from build123d import *

# Parameters (mm, degrees)
SKETCH1_R           = 25.4
BOSS_EXTRUDE1_DEPTH = 3.175
SKETCH2_R           = 12.7
SKETCH2_R_2         = 4.7625
BOSS_EXTRUDE2_DEPTH = 25.4
SKETCH3_R           = 3.175
CUT_EXTRUDE1_DEPTH  = 29.575


with BuildPart() as part:
    # Sketch1 → Boss-Extrude1 (new body)
    with BuildSketch(Plane(origin=(0, 0, 0), x_dir=(1, 0, 0), z_dir=(0, 1, 0))):
        Circle(SKETCH1_R)
    extrude(amount=BOSS_EXTRUDE1_DEPTH)

    # Sketch2 → Boss-Extrude2 (add)
    with BuildSketch(Plane(origin=(0, 3.175, 0), x_dir=(1, 0, 0), z_dir=(0, 1, 0))):
        Circle(SKETCH2_R)
        Circle(SKETCH2_R_2, mode=Mode.SUBTRACT)
    extrude(amount=BOSS_EXTRUDE2_DEPTH)

    # Sketch3 → Cut-Extrude1 (cut, through all)
    with BuildSketch(Plane.XZ):
        with Locations((-12.7, 12.7)):
            Circle(SKETCH3_R)
        with Locations((12.7, 12.7)):
            Circle(SKETCH3_R)
        with Locations((12.7, -12.7)):
            Circle(SKETCH3_R)
        with Locations((-12.7, -12.7)):
            Circle(SKETCH3_R)
    extrude(amount=-CUT_EXTRUDE1_DEPTH, mode=Mode.SUBTRACT)


solid = part.part
Verification items for the finished model (mm, model axes). A direction names the side the tool comes from. Coordinates: 2 decimals unless noted, no trailing zeros. Order: outer loops, then holes, each group sorted by start corner. A loop starts at its lowest first (then second) coordinate and runs counter-clockwise, first axis right, second up. Notation, with made-up numbers: M 15,63 L 34,63 A5 cw 34,68 Z; hole C -26.5,66.25 d1. An arc over 180 degrees is marked long. One line per item, written item: value. Start each with the question number.
Item 1: Sectioned sample at B-B on z = 15. Record the cut outline in (x, y) (3 decimals).
Item 2: Depth check by flat-ended pin: P1, Ø1, axis at x = -5, y = 19, coming from the +Z side; P2, Ø3, axis at x = 8, y = 5.5, coming from the +Z side; P3, Ø5, axis at x = 12.7, z = -12.7, coming from the -Y side; P4, Ø4, axis at y = 23.5, z = 7, coming from the -X side. Enter the tip coordinate at first touch or a pass-through.
Item 3: Sectioned sample at C-C on x = 0. Record the cut outline in (y, z) (1 decimal).
Item 4: Sectioned sample at A-A on x = 12. Record the cut outline in (y, z) (3 decimals).
Item 5: Access from +Z, -Z, +X, -X, +Y, -Y to the whole of each face (thin tool, end or side, straight path). Record for faces 1 (the flat face through (0, 3.175, 0)), 2 (the flat face through (5, 28.575, 0)).
Item 6: Thickness scan on probe 1 along X at (y, z) = (19.5, 0); probe 2 along Z at (x, y) = (-12.7, 1.2) (3 decimals); probe 3 along X at (y, z) = (3, -10). Record the ranges inside material, lowest first.
Item 7: Sectioned sample at D-D on y = 10.5. Record the cut outline in (x, z) (1 decimal), then the cut area to 3 significant figures.
Item 8: Mould release check, pull along Z, two halves, no side actions. Record for faces 3 (the flat face through (0, 0, 0)), 4 (the cylindrical face through (-5.506, 1.565, 24.796)), 5 (the cylindrical face through (10.18, 1.57, 10.77)): pulls with the +Z half, pulls with the -Z half, needs draft (parallel to the pull), parting line crosses it, or undercut.
Calculated:
1. outline: M -20.498,0 L -14.889,0 L -14.889,3.175 L -20.498,3.175 Z; M -10.511,0 L 10.511,0 L 10.511,3.175 L -10.511,3.175 Z; M 14.889,0 L 20.498,0 L 20.498,3.175 L 14.889,3.175 Z
2. P1: z = 11.88
2. P2: z = 10.91
2. P3: through
2. P4: x = -11.67
3. outline: M 0,-25.4 L 3.2,-25.4 L 3.2,-12.7 L 28.6,-12.7 L 28.6,-4.8 L 3.2,-4.8 L 3.2,4.8 L 28.6,4.8 L 28.6,12.7 L 3.2,12.7 L 3.2,25.4 L 0,25.4 Z
4. outline: M 0,-22.387 L 3.175,-22.387 L 3.175,-15.797 L 0,-15.797 Z; M 0,-9.603 L 3.175,-9.603 L 3.175,-4.158 L 28.575,-4.158 L 28.575,4.158 L 3.175,4.158 L 3.175,9.603 L 0,9.603 Z; M 0,15.797 L 3.175,15.797 L 3.175,22.387 L 0,22.387 Z
5. face 1: +Y
5. face 2: +Z, -Z, +X, -X, +Y
6. probe 1: -12.7 to -4.76, 4.76 to 12.7
6. probe 2: -21.997 to -15.875, -9.525 to 9.525, 15.875 to 21.997
6. probe 3: -23.35 to -14.37, -11.03 to 11.03, 14.37 to 23.35
7. outline: C 0,0 d25.4; hole C 0,0 d9.5
7. area: 435 mm^2
8. face 3: needs draft
8. face 4: parting line crosses it
8. face 5: undercut
